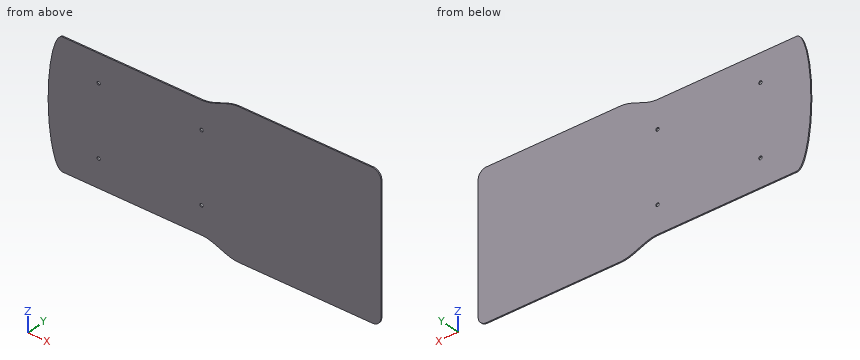
from build123d import *

# Parameters (mm, degrees)
SKETCH_1_W          = 278
SKETCH_1_H          = 120
EXTRUDE_1_DEPTH     = 1
SKETCH_2_W          = 129
SKETCH_2_H          = 8
CUT_EXTRUDE_1_DEPTH = 1
CUT_EXTRUDE_2_DEPTH = 1
CUT_EXTRUDE_4_DEPTH = 1
CUT_EXTRUDE_5_DEPTH = 1
SKETCH_16_R         = 1.39979
CUT_EXTRUDE_9_DEPTH = 10


with BuildPart() as part:
    # 스케치1 → 보스-돌출1 (new body)
    with BuildSketch(Plane(origin=(0, 0, 0), x_dir=(1, 0, 0), z_dir=(0, 1, 0))):
        Rectangle(SKETCH_1_W, SKETCH_1_H)
    extrude(amount=EXTRUDE_1_DEPTH)

    # 스케치2 → 컷-돌출1 (cut)
    with BuildSketch(Plane(origin=(0, 1, 0), x_dir=(1, 0, 0), z_dir=(0, 1, 0))):
        with Locations((-74.5, -56)):
            Rectangle(SKETCH_2_W, SKETCH_2_H)
        with Locations((-74.5, 56)):
            Rectangle(SKETCH_2_W, SKETCH_2_H)
    extrude(amount=-CUT_EXTRUDE_1_DEPTH, mode=Mode.SUBTRACT)

    # 스케치3 → 컷-돌출2 (cut)
    with BuildSketch(Plane(origin=(0, 1, 0), x_dir=(1, 0, 0), z_dir=(0, 1, 0))):
        with BuildLine():
            add(Edge.make_bspline(
                [(-127, 52), (-139, 52), (-139, 0)],
                knots=[3.141592654, 3.141592654, 3.141592654, 4.71238898, 4.71238898, 4.71238898], degree=2, weights=[1, 0.707106781, 1]))
            Line((-127, 52), (-139, 52))
            Line((-139, 52), (-139, 0))
        make_face()
        with BuildLine():
            Line((-139, -52), (-127, -52))
            add(Edge.make_bspline(
                [(-139, 0), (-139, -52), (-127, -52)],
                knots=[4.71238898, 4.71238898, 4.71238898, 6.283185307, 6.283185307, 6.283185307], degree=2, weights=[1, 0.707106781, 1]))
            Line((-139, 0), (-139, -52))
        make_face()
    extrude(amount=-CUT_EXTRUDE_2_DEPTH, mode=Mode.SUBTRACT)

    # 스케치4 → 컷-돌출4 (cut)
    with BuildSketch(Plane(origin=(0, 1, 0), x_dir=(1, 0, 0), z_dir=(0, 1, 0))):
        with BuildLine():
            Line((-10, 52), (-10, 60))
            Line((-10, 60), (20, 60))
            add(Edge.make_bspline(
                [(-10, 52), (0.64121866, 52.367223255), (9.376693721, 59.919927591), (20, 60)],
                knots=[0, 0, 0, 0, 1, 1, 1, 1], degree=3))
        make_face()
        with BuildLine():
            Line((-10, -52), (-10, -60))
            Line((-10, -60), (20, -60))
            add(Edge.make_bspline(
                [(-10, -52), (0.64121866, -52.367223255), (9.376693721, -59.919927591), (20, -60)],
                knots=[0, 0, 0, 0, 1, 1, 1, 1], degree=3))
        make_face()
    extrude(amount=-CUT_EXTRUDE_4_DEPTH, mode=Mode.SUBTRACT)

    # 스케치5 → 컷-돌출5 (cut)
    with BuildSketch(Plane(origin=(0, 1, 0), x_dir=(1, 0, 0), z_dir=(0, 1, 0))):
        with BuildLine():
            Line((132, 60), (139, 60))
            Line((139, 60), (139, 53))
            ThreePointArc((139, 53), (136.949747468, 57.949747468), (132, 60))
        make_face()
        with BuildLine():
            Line((139, -60), (139, -53))
            ThreePointArc((139, -53), (136.949747468, -57.949747468), (132, -60))
            Line((132, -60), (139, -60))
        make_face()
    extrude(amount=-CUT_EXTRUDE_5_DEPTH, mode=Mode.SUBTRACT)

    # 스케치16 → 컷-돌출9 (cut)
    with BuildSketch(Plane(origin=(0, 1, 0), x_dir=(1, 0, 0), z_dir=(0, 1, 0))):
        with Locations(Location((-96.85129, 29.0311, 0), (0, 0, 270))):
            Circle(SKETCH_16_R)
        with Locations(Location((-96.85109, -28.96802, 0), (0, 0, 270))):
            Circle(SKETCH_16_R)
        with Locations(Location((-10.85223, 29.03265, 0), (0, 0, 270))):
            Circle(SKETCH_16_R)
        with Locations(Location((-10.8511, -28.96784, 0), (0, 0, 270))):
            Circle(SKETCH_16_R)
    extrude(amount=-CUT_EXTRUDE_9_DEPTH, mode=Mode.SUBTRACT)


solid = part.part
Source: CAD feature listing. Evaluate the final solid. Frame: model axes, mm. Coordinates: 2 decimals unless noted, no trailing zeros. Order: outer loops, then holes, each group sorted by start corner. A loop starts at its lowest first (then second) coordinate and runs counter-clockwise, first axis right, second up. Notation, with made-up numbers: M 44,-15 L 76,-15 A33 ccw 76,17 Z; hole C 11.25,20.5 d3. An arc over 180 degrees is marked long. Write each question's results on one line, items separated by ' | '. Start each with the question number.
1. Section B-B, the plane y = 0.55. State how many separate pieces and enclosed holes the cut face has, then the cut area to 3 significant figures.
2. Material intervals for L1, parallel to X at y = 0.9, z = 28; L2, parallel to X at y = 0.45, z = -29.5; L3, parallel to Z at x = -77.5, y = 0.9, sorted ascending.
3. Pin query (flat end, axial travel): pin 1 (3 mm diameter, centred on x = -10.85, z = 28.97, fed in from +Y); pin 2 (0.5 mm diameter, centred on x = -93, y = 0.5, fed in from -Z). Return the tip coordinate at first contact, or that it passes through.
4. Section A-A, the plane x = -33. Return the cut outline in (y, z), then the cut area to 3 significant figures.
Solution:
1) separate pieces: 1 | enclosed holes: 4 | area: 30,700 mm²
2) L1: -137.11 to -97.86, -95.84 to -11.86, -9.84 to 139 | L2: -136.88 to -98.17, -95.53 to -12.17, -9.53 to 139 | L3: -52 to 52
3) pin 1: y = 1 | pin 2: z = -52
4) outline: M 0,-52 L 1,-52 L 1,52 L 0,52 Z | area: 104 mm²
